Here's how the part is built. I have some questions about the finished solid (model axes, mm). A direction names the side the tool comes from. Coordinates: 2 decimals unless noted, no trailing zeros. Write each loop counter-clockwise with the first axis right and the second up, starting at its lowest first coordinate (ties: lowest second). Pieces come first, ordered by that corner, then holes. Notation, with made-up numbers: M 89,-12 L 94,-12 A25 cw 94,3 Z; hole C -13,-31.5 d2. An arc over 180 degrees is marked long. Use a Markdown table: item, result.
```python
from build123d import *

# Parameters (mm, degrees)
SKETCH1_R           = 22.225
BOSS_EXTRUDE1_DEPTH = 25.4
SKETCH2_R           = 16.891
BOSS_EXTRUDE2_DEPTH = 25.4
SKETCH3_R           = 15.621
CUT_EXTRUDE1_DEPTH  = 50.8
SKETCH4_R           = 19.685
CUT_EXTRUDE2_DEPTH  = 22.225


with BuildPart() as part:
    # Sketch1 → Boss-Extrude1 (new body)
    with BuildSketch(Plane.XY):
        Circle(SKETCH1_R)
    extrude(amount=BOSS_EXTRUDE1_DEPTH)

    # Sketch2 → Boss-Extrude2 (add)
    with BuildSketch(Plane.XY.offset(25.4)):
        Circle(SKETCH2_R)
    extrude(amount=BOSS_EXTRUDE2_DEPTH)

    # Sketch3 → Cut-Extrude1 (cut)
    with BuildSketch(Plane.XY.offset(50.8)):
        Circle(SKETCH3_R)
    extrude(amount=-CUT_EXTRUDE1_DEPTH, mode=Mode.SUBTRACT)

    # Sketch4 → Cut-Extrude2 (cut)
    with BuildSketch(Plane(origin=(0, 0, 0), x_dir=(-1, 0, 0), z_dir=(0, 0, -1))):
        Circle(SKETCH4_R)
    extrude(amount=-CUT_EXTRUDE2_DEPTH, mode=Mode.SUBTRACT)


solid = part.part
```
1. Suppose I cut it at C-C on z = 36. Write out the boundary of the cut face in (x, y).
Answers follow:
| item | result |
|---|---|
| outline | C 0,0 d33.78; hole C 0,0 d31.24 |
2. Will these pins go through, and if not, where does the flat tip stop? pin 1 Ø2 at (x, z) = (13.5, 17) entering from +Y; pin 2 Ø3 at (x, y) = (14.5, 13) entering from +Z; pin 3 Ø5 at (y, z) = (4, 33.5) entering from -X; pin 4 Ø8 at (x, y) = (-0.5, -10) entering from +Z.
Answers follow:
| item | result |
|---|---|
| pin 1 | stops at y = 18.38 |
| pin 2 | stops at z = 25.4 |
| pin 3 | stops at x = -16.82 |
| pin 4 | passes through |
3. Suppose I cut it at D-D on z = 20. Write out the boundary of the cut face in (x, y) (3 decimals).
Answers follow:
| item | result |
|---|---|
| outline | C 0,0 d44.45; hole C 0,0 d39.37 |
4. Suppose I cut it at A-A on x = 0. Write out the boundary of the cut face in (y, z) (3 decimals).
Answers follow:
| item | result |
|---|---|
| outline | M -22.225,0 L -19.685,0 L -19.685,22.225 L -15.621,22.225 L -15.621,50.8 L -16.891,50.8 L -16.891,25.4 L -22.225,25.4 Z; M 15.621,22.225 L 19.685,22.225 L 19.685,0 L 22.225,0 L 22.225,25.4 L 16.891,25.4 L 16.891,50.8 L 15.621,50.8 Z |
5. Which directions (+Z, -Z, +X, -X, +Y, -Y) give clear straight access to the entire face, cutting with the end or side of a thin tool? Please do faces 1 (the face through (16.111, 5.074, 37.922)), 2 (the face through (15.62, -11.98, 10.96)), 3 (the face through (-2, -20, 0)).
Answers follow:
| item | result |
|---|---|
| face 1 | +Z |
| face 2 | -Z |
| face 3 | -Z, +X, -X, +Y, -Y |
6. We'd pull the mould along X, two halves only. Please class faces 4 (the face through (-2.03, 15.49, 36.71)), 5 (the face through (6, 15, 22.225)), 6 (the face through (21.199, 6.676, 12.522)), 7 (the face through (15, -5, 50.8)): +X half, -X half, draft (parallel to the pull), parting line (faces both ways), or undercut.
Answers follow:
| item | result |
|---|---|
| face 4 | undercut |
| face 5 | undercut |
| face 6 | parting line |
| face 7 | draft |
7. I need wall thicknesses on probe 1 along Y at (x, z) = (0, 17) (3 decimals); probe 2 along X at (y, z) = (-0.5, 38.5); probe 3 along Z at (x, y) = (17, -1.5) (3 decimals). Which ranges of each line are inside material? Lowest first, please.
Answers follow:
| item | result |
|---|---|
| probe 1 | y = -22.225 to -19.685, 19.685 to 22.225 |
| probe 2 | x = -16.88 to -15.61, 15.61 to 16.88 |
| probe 3 | z = 22.225 to 25.4 |
